```python
from build123d import *

# Parameters (mm, degrees)
F1_DEPTH = 3.175


# Not quite as in the source:
# - a feature names something its author has since deleted; it is built from what else it names


with BuildPart() as f1:
    # F0 (on Front) → F1 (new body)
    with BuildSketch(Plane.XZ):
        with BuildLine():
            ThreePointArc((-19.05, 0), (-18.7565324084, 3.330914591), (-17.8851714423, 6.5592028846))
            ThreePointArc((-17.8851714423, 6.5592028846), (-21.3208303202, 6.2628506055), (-24.1480220477, 4.2883725643))
            ThreePointArc((-24.1480220477, 4.2883725643), (-22.1735440066, 1.4611808368), (-19.05, 0))
        make_face()
        with BuildLine():
            ThreePointArc((17.9570302857, -6.3598398815), (18.774769332, -3.2265363052), (19.05, 0))
            ThreePointArc((19.05, 0), (3.330914591, 18.7565324084), (-17.8851714423, 6.5592028846))
            ThreePointArc((-17.8851714423, 6.5592028846), (-18.7565324084, 3.330914591), (-19.05, 0))
            ThreePointArc((-19.05, 0), (-18.9787164623, -1.6464572402), (-18.7653993235, -3.2805926645))
            ThreePointArc((-18.7653993235, -3.2805926645), (-17.902768373, -6.5110202414), (-16.4886138833, -9.5408653804))
            ThreePointArc((-16.4886138833, -9.5408653804), (-15.5953963885, -10.940114784), (-14.5837536932, -12.2562893331))
            ThreePointArc((-14.5837536932, -12.2562893331), (-12.2164908848, -14.6171081429), (-9.4729601013, -16.5277199552))
            ThreePointArc((-9.4729601013, -16.5277199552), (-7.9923386115, -17.2923400244), (-6.4505607615, -17.9246413036))
            ThreePointArc((-6.4505607615, -17.9246413036), (-3.2177031841, -18.7762852082), (0.114253165, -19.0496573779))
            ThreePointArc((0.114253165, -19.0496573779), (1.7773096461, -18.9669098807), (3.4267873399, -18.7392536812))
            ThreePointArc((3.4267873399, -18.7392536812), (6.6502136181, -17.8515309941), (9.6687925813, -16.4139254909))
            ThreePointArc((9.6687925813, -16.4139254909), (11.058239811, -15.5118610193), (12.3640641678, -14.4924952045))
            ThreePointArc((12.3640641678, -14.4924952045), (14.707623832, -12.107365577), (16.5980379903, -9.3492050396))
            ThreePointArc((16.5980379903, -9.3492050396), (17.3420662524, -7.8838593403), (17.9570302857, -6.3598398815))
        make_face()
        with BuildLine():
            ThreePointArc((-16.4886138833, -9.5408653804), (-17.902768373, -6.5110202414), (-18.7653993235, -3.2805926645))
            ThreePointArc((-18.7653993235, -3.2805926645), (-21.5590287963, -5.2571672852), (-23.0027619685, -8.3598834163))
            ThreePointArc((-23.0027619685, -8.3598834163), (-19.9027732819, -9.816837479), (-16.4886138833, -9.5408653804))
        make_face()
        with BuildLine():
            ThreePointArc((-9.4729601013, -16.5277199552), (-12.2164908848, -14.6171081429), (-14.5837536932, -12.2562893331))
            ThreePointArc((-14.5837536932, -12.2562893331), (-15.9914516234, -15.352990661), (-15.6868096556, -18.7409643694))
            ThreePointArc((-15.6868096556, -18.7409643694), (-12.286729337, -18.4573983143), (-9.4729601013, -16.5277199552))
        make_face()
        with BuildLine():
            ThreePointArc((-4.1604686233, -24.0732680372), (-1.3577089131, -22.1276679749), (0.114253165, -19.0496573779))
            ThreePointArc((0.114253165, -19.0496573779), (-3.2177031841, -18.7762852082), (-6.4505607615, -17.9246413036))
            ThreePointArc((-6.4505607615, -17.9246413036), (-6.1149672512, -21.3004400299), (-4.1604686233, -24.0732680372))
        make_face()
        with BuildLine():
            ThreePointArc((8.4877873574, -22.928007958), (9.9447352105, -19.8280535223), (9.6687925813, -16.4139254909))
            ThreePointArc((9.6687925813, -16.4139254909), (6.6502136181, -17.8515309941), (3.4267873399, -18.7392536812))
            ThreePointArc((3.4267873399, -18.7392536812), (5.4050438072, -21.50087086), (8.4877873574, -22.928007958))
        make_face()
        with BuildLine():
            ThreePointArc((18.8688683105, -15.6120556451), (18.5725160314, -12.1763967671), (16.5980379903, -9.3492050396))
            ThreePointArc((16.5980379903, -9.3492050396), (14.707623832, -12.107365577), (12.3640641678, -14.4924952045))
            ThreePointArc((12.3640641678, -14.4924952045), (15.4680658678, -15.9145025235), (18.8688683105, -15.6120556451))
        make_face()
    extrude(amount=F1_DEPTH)


solid = f1.part
```
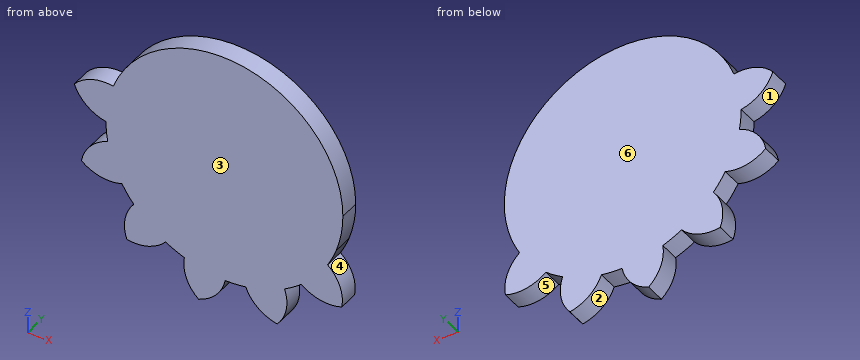
Design review of the part built by this model. Coordinates are the model's own, in mm. Face numbers are marked on the shaded views. A direction names the side the tool comes from. Coordinates: 2 decimals unless noted, no trailing zeros. Order: outer loops, then holes, each group sorted by start corner. A loop starts at its lowest first (then second) coordinate and runs counter-clockwise, first axis right, second up. Notation, with made-up numbers: M 26.25,0 L 56.25,0 A25 ccw 56.25,17 Z; hole C 42,24 d3. An arc over 180 degrees is marked long. Answer as a JSON object with one key per item and string values. Group by question number.
1) Wall thickness on L1, parallel to Z at x = -20.5, y = -0.6; L2, parallel to X at y = -1.1, z = -0.5; L3, parallel to X at y = -0.4, z = -19.5: over which ranges is each line inside the solid? List them lowest first.
2) Add section C-C, the plane x = -14. Write out the cut boundary in (y, z) (3 decimals), then the cut area to 3 significant figures.
3) Tool access review of the marked faces 1, 2 and 3: name each direction out of +Z, -Z, +X, -X, +Y, -Y from which nothing blocks a thin tool from reaching the whole face with its end or side.
4) Add section A-A, the plane y = -1.7. Write out the cut boundary in (x, z), then the cut area to 3 significant figures.
5) For pin 1 (8 mm diameter, centred on x = 5.5, z = 3.5, fed in from +Y); pin 2 (2 mm diameter, centred on x = -16.5, z = 13.5, fed in from +Y), all flat-tipped, find the tip position at first contact; note any pin that passes through.
6) Add section B-B, the plane z = -7. Write out the cut boundary in (x, y) (3 decimals).
7) Mouldability with a two-part tool opening along Z and no side actions: class the marked faces 4, 5 and 6 as pulls with the +Z half, pulls with the -Z half, needs draft (parallel to the pull), parting line crosses it, or undercut.
Computed values:
{
 "1": {"L1": "z = -9.68 to -4.24, 0.43 to 6.5", "L2": "x = -19.04 to 19.04", "L3": "x = -6.51 to 0.01, 3.77 to 10"},
 "2": {"outline": "M -3.175,-18.823 L 0,-18.823 L 0,12.919 L -3.175,12.919 Z", "area": "101 mm^2"},
 "3": {"face 1": "-X, +Y, -Y", "face 2": "-Z, +Y, -Y", "face 3": "+Z, -Z, +X, -X, -Y"},
 "4": {"outline": "M -24.15,4.29 A6.66 ccw -19.05,0 A19.05 ccw -18.77,-3.28 A6.66 ccw -23,-8.36 A6.66 ccw -16.49,-9.54 A19.05 ccw -14.58,-12.26 A6.66 ccw -15.69,-18.74 A6.66 ccw -9.47,-16.53 A19.05 ccw -6.45,-17.92 A6.66 ccw -4.16,-24.07 A6.66 ccw 0.11,-19.05 A19.05 ccw 3.43,-18.74 A6.66 ccw 8.49,-22.93 A6.66 ccw 9.67,-16.41 A19.05 ccw 12.36,-14.49 A6.66 ccw 18.87,-15.61 A6.66 ccw 16.6,-9.35 A19.05 ccw long -17.89,6.56 A6.66 ccw Z", "area": "1,290 mm^2"},
 "5": {"pin 1": "stops at y = 0", "pin 2": "passes through"},
 "6": {"outline": "M -22.608,-3.175 L 17.717,-3.175 L 17.717,0 L -22.608,0 Z"},
 "7": {"face 4": "undercut", "face 5": "pulls with the -Z half", "face 6": "needs draft"}
}
